Geometry: final body of the model. Coordinates: model frame, mm. A direction names the side the tool comes from. Give positions to 0.01 mm unless a question says otherwise; leave off trailing zeros. Loops run counter-clockwise (first coordinate to the right, second up) from the corner with the lowest first, then second, coordinate; pieces in that order, holes last. Notation, with made-up numbers: (67.5, -18.75) - (101.5, -18.75) arc R20 ccw to (101.5, 11.25) - close; hole circle Ø5 at (63.5, -6.5). An arc over 180 degrees is marked (long way). Answer in a Markdown table with one row per item.
from build123d import *

# Parameters (mm, degrees)
EXTRUDE_1_DEPTH     = 5
EXTRUDE_2_DEPTH     = 51
CUT_EXTRUDE_1_DEPTH = 10


with BuildPart() as part:
    # Sketch 1 → Extrude 1 (new body)
    with BuildSketch(Plane.XY):
        Polygon((20, -25), (20, 0), (20, 25), (-25, 25), (-25, -25), align=None)
        with BuildLine():
            ThreePointArc((8, 0), (9.5, 1.5), (11, 0))
            ThreePointArc((11, 0), (9.5, -1.5), (8, 0))
        make_face(mode=Mode.SUBTRACT)
    extrude(amount=EXTRUDE_1_DEPTH)

    # Sketch 1_4 → Extrude 2 (add)
    with BuildSketch(Plane.XY):
        Polygon((20, 25), (20, 0), (20, -25), (25, -25), (25, 25), align=None)
    extrude(amount=EXTRUDE_2_DEPTH)

    # Sketch 2 → Cut-Extrude 1 (cut)
    with BuildSketch(Plane.ZY.offset(-20)):
        with BuildLine():
            ThreePointArc((20, 0), (21.5, -1.5), (23, 0))
            Line((23, 0), (20, 0))
        make_face()
        with BuildLine():
            Line((20, 0), (23, 0))
            ThreePointArc((23, 0), (21.5, 1.5), (20, 0))
        make_face()
    extrude(amount=-CUT_EXTRUDE_1_DEPTH, mode=Mode.SUBTRACT)


solid = part.part
Q1. Material intervals for line 1 along Y through (x, z) = (22.35, 21.5); line 2 along Z through (x, y) = (-10, -5.5); line 3 along X through (y, z) = (18.5, 23.5), sorted ascending.
Check values:
| item | result |
|---|---|
| line 1 | -25 to -1.5, 1.5 to 25 |
| line 2 | 0 to 5 |
| line 3 | 20 to 25 |
Q2. Cut plane A-A (z = 21.5). Output: boundary loops of the cut face in (x, y).
Check values:
| item | result |
|---|---|
| outline | (20, -25) - (25, -25) - (25, -1.5) - (20, -1.5) - close; (20, 1.5) - (25, 1.5) - (25, 25) - (20, 25) - close |
Q3. Reachability of faces 5 (the flat face through (20, 0, 28)), 6 (the flat face through (20.3, -25, 15.9)) from +Z, -Z, +X, -X, +Y, -Y: full face, straight path, thin tool, end or side. Return the list, or none.
Check values:
| item | result |
|---|---|
| face 5 | +Z, -X, +Y, -Y |
| face 6 | +Z, -Z, +X, -X, -Y |
Q4. Cut plane D-D (z = 47). Output: boundary loops of the cut face in (x, y).
Check values:
| item | result |
|---|---|
| outline | (20, -25) - (25, -25) - (25, 25) - (20, 25) - close |
Q5. First-contact query: pin 1 (2 mm diameter, centred on x = 6, y = -17, fed in from -Z); pin 2 (8 mm diameter, centred on x = 5, y = -14.5, fed in from +Z). Flat tips, straight axial feed; report the tip coordinate or a pass-through.
Check values:
| item | result |
|---|---|
| pin 1 | z = 0 |
| pin 2 | z = 5 |
Q6. Cut plane C-C (x = 9.5). Output: boundary loops of the cut face in (y, z), and give its area (3 significant figures).
Check values:
| item | result |
|---|---|
| outline | (-25, 0) - (-1.5, 0) - (-1.5, 5) - (-25, 5) - close; (1.5, 0) - (25, 0) - (25, 5) - (1.5, 5) - close |
| area | 235 mm² |
Q7. Draft query along Z for faces 1 (the cylindrical face through (22, 0, 20)), 2 (the cylindrical face through (8, 0, 2)), 3 (the flat face through (0, 0, 0)), 4 (the flat face through (22, 0, 51)). Return one class per face: pulls with the +Z half, pulls with the -Z half, needs draft (parallel to the pull), parting line crosses it, or undercut.
Check values:
| item | result |
|---|---|
| face 1 | undercut |
| face 2 | needs draft |
| face 3 | pulls with the -Z half |
| face 4 | pulls with the +Z half |
Q8. Cut plane B-B (y = 0). Output: boundary loops of the cut face in (x, z).
Check values:
| item | result |
|---|---|
| outline | (-25, 0) - (8, 0) - (8, 5) - (-25, 5) - close; (11, 0) - (25, 0) - (25, 20) - (20, 20) - (20, 5) - (11, 5) - close; (20, 23) - (25, 23) - (25, 51) - (20, 51) - close |
